Work out the finished part from the listing and answer in its coordinate system (mm). A direction names the side the tool comes from. Give positions to 0.01 mm unless a question says otherwise; leave off trailing zeros. Write each loop counter-clockwise with the first axis right and the second up, starting at its lowest first coordinate (ties: lowest second). Pieces come first, ordered by that corner, then holes.
1) Given pin 1 Ø12 at (x, z) = (30.5, -7.5) entering from -Y; pin 2 Ø12 at (x, z) = (-2, -6.5) entering from -Y; pin 3 Ø0.7 at (x, y) = (-11, -0.5) entering from +Z, each flat-ended and moving along its own axis, determine where each tip first touches the part or whether it passes through.
2) A tool of negligible diameter and unlimited length cuts with its end or side. For faces 1 (the face through (-2.031, -3.244, -0.72)), 2 (the face through (-11.028, 1.724, -1.014)), 3 (the face through (29.14, -9.76, -2.17)), from which of +Z, -Z, +X, -X, +Y, -Y can it reach the whole face along a straight path? Write none if from no direction.
3) Find section A-A (x = 15.5). Determine the outline of the cut face in (y, z).
4) Determine the mould class of faces 4 (the face through (39, 0, 0)), 5 (the face through (-11.028, -1.724, 1.014)), 6 (the face through (-1, 1.2, -3.3)) for opening direction X: pulls with the +X half, pulls with the -X half, needs draft (parallel to the pull), parting line crosses it, or undercut.
5) Straight lines are drawn through the part: probe 1 along X at (y, z) = (-5.25, 1); probe 2 along X at (y, z) = (1.25, -0.75); probe 3 along Z at (x, y) = (35.5, 0.25). For each, find the intervals that lie inside material, in ascending order.
```python
from build123d import *

# Parameters (mm, degrees)
CUT_EXTRUDE_1_DEPTH = 4


with BuildPart() as part:
    # Sketch 1 → Revolve 1 (revolve)
    with BuildSketch(Plane.XY, mode=Mode.PRIVATE) as revolve_1_sk:
        Polygon((-13, 0), (-13, 3.233), (-12.233, 4), (-3.767, 4), (-3.0905, 3.3235), (-1, 3.3235), (-1, 5), (0, 5), (0, 8.5), (19, 10), (39, 10), (39, 0), align=None)
    revolve(revolve_1_sk.sketch.rotate(Axis((39, 0, 0), (-1, 0, 0)), 270), axis=Axis((39, 0, 0), (-1, 0, 0)))

    # Sketch 2 → Cut-Extrude 1 (cut)
    with BuildSketch(Plane(origin=(-13, 0, 0), x_dir=(0, 0, -1), z_dir=(1, 0, 0))):
        Polygon((-2, 1.154700538), (-2, -1.154700538), (0, -2.309401077), (2, -1.154700538), (2, 1.154700538), (0, 2.309401077), align=None)
    extrude(amount=CUT_EXTRUDE_1_DEPTH, mode=Mode.SUBTRACT)

    # Sketch 3 → Cut-Revolve 1 (revolve, cut)
    with BuildSketch(Plane.XY, mode=Mode.PRIVATE) as cut_revolve_1_sk:
        Polygon((-9, 0), (-9, 2.309401077), (-7.67, 0), align=None)
    revolve(cut_revolve_1_sk.sketch.rotate(Axis((-7.67, 0, 0), (-1, 0, 0)), 270), axis=Axis((-7.67, 0, 0), (-1, 0, 0)), mode=Mode.SUBTRACT)


solid = part.part
```
Results:
1. pin 1: stops at y = -9.89
1. pin 2: stops at y = -8.48
1. pin 3: stops at z = 4
2. face 1: none
2. face 2: -X
2. face 3: +X, -X
3. outline: circle Ø19.45 at (0, 0)
4. face 4: pulls with the +X half
4. face 5: needs draft
4. face 6: undercut
5. probe 1: x = 0 to 39
5. probe 2: x = -8.51 to 39
5. probe 3: z = -10 to 10
